Build history of the part. All positions in model axes, mm. A direction names the side the tool comes from. Round coordinates to 2 decimals unless told otherwise and drop trailing zeros. Write each loop counter-clockwise with the first axis right and the second up, starting at its lowest first coordinate (ties: lowest second). Pieces come first, ordered by that corner, then holes. Notation, with made-up numbers: M 72.25,12 L 103.25,12 A25 ccw 103.25,38 Z; hole C -15.75,-25.5 d11. An arc over 180 degrees is marked long. Write item = value, one per line. Start each with the question number.
Q1. Pull direction Z, two halves, no side cores. Call faces 1 (the flat face through (-13, 4, 33)), 2 (the flat face through (9.1, 10, 1)), 3 (the flat face through (0, 0, 35)), 4 (the flat face through (-10.76, 3.64, 9.986)): released by +Z, released by -Z, zero draft, split by the parting line, or undercut.
Q2. Drop a flat-ended pin along its axis: P1, Ø6.5, axis at x = -10, z = 18.5, coming from the +Y side. Give the stop position or say it passes through.
Q3. Band-saw the part on B-B on x = -4. Write the cut outline in (y, z).
Q4. Tool access for faces 5 (the flat face through (2, 3, 33)), 6 (the cylindrical face through (-15.43, 12.9, 10.01)), 7 (the cylindrical face through (12.7, -0.7, 21)), 8 (the flat face through (-9.1, -1, 1)): list every direction of +Z, -Z, +X, -X, +Y, -Y with a clear straight run to the whole face (end or side of a thin tool).
Q5. Band-saw the part on A-A on z = 6. Write the cut outline in (x, y).
Q6. Band-saw the part on C-C on z = 17.75. Write the cut outline in (x, y) (3 decimals), plus the area to 3 significant figures.
Q7. Probe L1, parallel to Z at x = 12.15, y = 0 (3 decimals); L2, parallel to Z at x = 15.2, y = 0; L3, parallel to Z at x = -9.5, y = 0.75. List the from-to ranges inside material, lowest first.
```python
from build123d import *

# Parameters (mm, degrees)
SKETCH1_W               = 32
SKETCH1_H               = 27
BOSS_EXTRUDE1_DEPTH     = 35
FILLET1_R               = 2
CUT_EXTRUDE1_DEPTH      = 1
CUT_EXTRUDE1_DEPTH_BACK = 28
BOSS_EXTRUDE2_DEPTH     = 7
BOSS_EXTRUDE3_DEPTH     = 1.8
SKETCH5_W               = 2
SKETCH5_H               = 7
CUT_EXTRUDE2_DEPTH      = 33
CUT_EXTRUDE3_DEPTH      = 20
SKETCH7_W               = 2
SKETCH7_H               = 33
BOSS_EXTRUDE4_DEPTH     = 0.25
FILLET2_R               = 6
CUT_EXTRUDE5_DEPTH      = 4.5
SKETCH14_W              = 2.5
SKETCH14_H              = 20
CUT_EXTRUDE6_DEPTH      = 20
SKETCH16_W              = 2
SKETCH16_H              = 4
SKETCH16_H_2            = 2
BOSS_EXTRUDE5_DEPTH     = 20
BOSS_EXTRUDE6_DEPTH     = 20


with BuildPart() as part:
    # Sketch1 → Boss-Extrude1 (new body)
    with BuildSketch(Plane.XY):
        Rectangle(SKETCH1_W, SKETCH1_H)
    extrude(amount=BOSS_EXTRUDE1_DEPTH)

    # Fillet1
    fillet1_edges = [part.edges().sort_by_distance(p)[0] for p in [
        (16, -13.5, 17.5),
        (-16, -13.5, 17.5),
        (-16, 13.5, 17.5),
        (16, 13.5, 17.5),
    ]]
    fillet(fillet1_edges, radius=FILLET1_R)

    # Sketch2 → Cut-Extrude1 (cut, two sides)
    with BuildSketch(Plane.XZ.offset(13.5)) as cut_extrude1_sk:
        Polygon((-9.1, 0), (-9.1, 1.8), (-11.1, 1.8), (-11.1, 5), (11.1, 5), (11.1, 1.8), (9.1, 1.8), (9.1, 0), align=None)
    extrude(amount=CUT_EXTRUDE1_DEPTH, mode=Mode.SUBTRACT)
    extrude(cut_extrude1_sk.sketch, amount=-CUT_EXTRUDE1_DEPTH_BACK, mode=Mode.SUBTRACT)

    # Sketch3 → Boss-Extrude2 (add)
    with BuildSketch(Plane.XZ.offset(13.5)):
        Polygon((-9.1, 0), (-9.1, 1.8), (-11.1, 1.8), (-11.1, 5), (11.1, 5), (11.1, 1.8), (9.1, 1.8), (9.1, 0), align=None)
    extrude(amount=-BOSS_EXTRUDE2_DEPTH)

    # Sketch4 → Boss-Extrude3 (add)
    with BuildSketch(Plane(origin=(0, 0, 1.8), x_dir=(-1, 0, 0), z_dir=(0, 0, -1))):
        with BuildLine():
            Line((-9.1, 6.5), (-9.1, 5.5))
            ThreePointArc((-9.1, 5.5), (-8.85, 6), (-9.1, 6.5))
        make_face()
    boss_extrude3 = extrude(amount=BOSS_EXTRUDE3_DEPTH)

    # Mirror1: Boss-Extrude3 across plane
    add(boss_extrude3.mirror(Plane(origin=(0, 0, 0), x_dir=(0, 0, 1), z_dir=(1, 0, 0))))

    # Sketch5 → Cut-Extrude2 (cut)
    with BuildSketch(Plane(origin=(0, 0, 0), x_dir=(-1, 0, 0), z_dir=(0, 0, -1))):
        with Locations((0, -10)):
            Rectangle(SKETCH5_W, SKETCH5_H)
    extrude(amount=-CUT_EXTRUDE2_DEPTH, mode=Mode.SUBTRACT)

    # Sketch6 → Cut-Extrude3 (cut)
    with BuildSketch(Plane(origin=(0, 13.5, 0), x_dir=(1, 0, 0), z_dir=(0, 1, 0))):
        Polygon((-12.5, -7.5), (-12.5, -9), (-11.5, -9), (-11.5, -33), (11.5, -33), (11.5, -9), (12.5, -9), (12.5, -7.5), align=None)
    extrude(amount=-CUT_EXTRUDE3_DEPTH, mode=Mode.SUBTRACT)

    # Sketch7 → Boss-Extrude4 (add)
    with BuildSketch(Plane.XZ.offset(13.5)):
        with Locations((0, 16.5)):
            Rectangle(SKETCH7_W, SKETCH7_H)
    extrude(amount=-BOSS_EXTRUDE4_DEPTH)

    # Fillet2
    fillet2_edges = [part.edges().sort_by_distance(p)[0] for p in [
        (0, -13.25, 33),
    ]]
    fillet(fillet2_edges, radius=FILLET2_R)

    # Sketch9 → Cut-Revolve1 (revolve, cut)
    with BuildSketch(Plane(origin=(0, 0, 17.75), x_dir=(-1, 0, 0), z_dir=(0, 0, -1))):
        Polygon((-15, 4.25), (-14, 4.25), (-14, 3.325), (-11.5, 3.325), (-11.5, 0), (-16, 0), (-16, 3.75), (-15, 3.75), align=None)
    revolve(axis=Axis((16, 0, 17.75), (-1, 0, 0)), mode=Mode.SUBTRACT)

    # Sketch11 → Cut-Extrude5 (cut)
    with BuildSketch(Plane(origin=(-16, 0, 44), x_dir=(0, 0, -1), z_dir=(1, 0, 0))):
        with BuildLine():
            Line((24.25, 23), (24.25, 0))
            ThreePointArc((24.25, 0), (21, -3.25), (17.75, 0))
            Line((17.75, 0), (17.75, 23))
            ThreePointArc((17.75, 23), (21, 26.25), (24.25, 23))
        make_face()
    extrude(amount=CUT_EXTRUDE5_DEPTH, mode=Mode.SUBTRACT)

    # Sketch14 → Cut-Extrude6 (cut)
    with BuildSketch(Plane(origin=(0, 13.5, 0), x_dir=(1, 0, 0), z_dir=(0, 1, 0))):
        with Locations((-12.75, -23)):
            Rectangle(SKETCH14_W, SKETCH14_H)
    extrude(amount=-CUT_EXTRUDE6_DEPTH, mode=Mode.SUBTRACT)

    # Sketch16 → Boss-Extrude5 (add)
    with BuildSketch(Plane(origin=(0, 13.5, 0), x_dir=(1, 0, 0), z_dir=(0, 1, 0))):
        with Locations((-11, -13)):
            Rectangle(SKETCH16_W, SKETCH16_H)
        with Locations((-11, -32)):
            Rectangle(SKETCH16_W, SKETCH16_H_2)
    extrude(amount=-BOSS_EXTRUDE5_DEPTH)

    # Sketch20 → Boss-Extrude6 (add)
    with BuildSketch(Plane(origin=(0, 13.5, 0), x_dir=(1, 0, 0), z_dir=(0, 1, 0))):
        Polygon((-11.5, -9), (-10, -11), (-11.5, -11), align=None)
        Polygon((-10, -31), (-8.5, -33), (-10, -33), align=None)
    extrude(amount=-BOSS_EXTRUDE6_DEPTH)


solid = part.part
```
Conclusion:
q1.face_1 = undercut
q1.face_2 = zero draft
q1.face_3 = released by +Z
q1.face_4 = undercut
q2.P1 = -6.5
q3.outline = M -13.5,0 L -6.5,0 L -6.5,5 L 13.5,5 L 13.5,7.5 L -6.5,7.5 L -6.5,33 L 13.5,33 L 13.5,35 L -13.5,35 Z
q4.face_5 = +Y
q4.face_6 = +Z, -Z, -X, +Y
q4.face_7 = +X
q4.face_8 = -Z
q5.outline = M -16,-11.5 A2 ccw -14,-13.5 L 14,-13.5 A2 ccw 16,-11.5 L 16,11.5 A2 ccw 14,13.5 L -14,13.5 A2 ccw -16,11.5 Z; hole M -1,-13.25 L 1,-13.25 L 1,-6.5 L -1,-6.5 Z
q6.outline = M -16,-11.5 A2 ccw -14,-13.5 L 14,-13.5 A2 ccw 16,-11.5 L 16,-3.75 L 15,-3.75 L 15,-4.25 L 14,-4.25 L 14,-3.325 L 11.5,-3.325 L 11.5,-6.5 L 1,-6.5 L 1,-13.25 L -1,-13.25 L -1,-6.5 L -14,-6.5 L -14,13.5 A2 ccw -16,11.5 Z; M 11.5,3.325 L 14,3.325 L 14,4.25 L 15,4.25 L 15,3.75 L 16,3.75 L 16,11.5 A2 ccw 14,13.5 L 11.5,13.5 Z
q6.area = 304 mm^2
q7.L1 = 0 to 7.5, 9 to 14.425, 21.075 to 35
q7.L2 = 0 to 14, 21.5 to 35
q7.L3 = 0 to 1.8, 5 to 7.5, 31.67 to 35
